```python
from build123d import *

# Parameters (mm, degrees)
SKETCH1_W              = 25.4
SKETCH1_H              = 12.7
BOSS_EXTRUDE1_DEPTH    = 4.7625
F_10_32_TAPPED_HOLE1_D = 4.0386
F_10_32_TAPPED_HOLE2_D = 4.0386


with BuildPart() as part:
    # Sketch1 → Boss-Extrude1 (new, symmetric)
    with BuildSketch(Plane(origin=(0, 0, 0), x_dir=(0, 0, -1), z_dir=(1, 0, 0))):
        Rectangle(SKETCH1_W, SKETCH1_H)
    extrude(amount=BOSS_EXTRUDE1_DEPTH, both=True)

    # #10-32 Tapped Hole1 (through all)
    with Locations(Plane(origin=(0, 6.35, 0), x_dir=(1, 0, 0), z_dir=(0, 1, 0))):
        with Locations((0, 0)):
            Hole(F_10_32_TAPPED_HOLE1_D / 2)

    # #10-32 Tapped Hole2 (through all)
    with Locations(Plane(origin=(4.7625, 0, 0), x_dir=(0, 0, -1), z_dir=(1, 0, 0))):
        with Locations((-7.62, 0), (7.62, 0)):
            Hole(F_10_32_TAPPED_HOLE2_D / 2)


solid = part.part
```
Geometry: final body of the model. Coordinates: model frame, mm. Give positions to 0.01 mm unless a question says otherwise; leave off trailing zeros. Write each loop counter-clockwise with the first axis right and the second up, starting at its lowest first coordinate (ties: lowest second). Pieces come first, ordered by that corner, then holes.
1. Draft query along Y for faces 1 (the flat face through (2.2, -6.35, 0.2)), 2 (the cylindrical face through (-0.067, 0.607, -5.694)), 3 (the flat face through (4.762, 0, 0)). Return one class per face: released by +Y, released by -Y, zero draft, split by the parting line, or undercut.
2. Section query C-C, the plane y = 0. Return loops of the section in (x, z).
3. Section query D-D, the plane z = 7.62. Return loops of the section in (x, y).
4. Line query: probe 1 along Y at (x, z) = (2.25, 7.62); probe 2 along Z at (x, y) = (-1.5, -1); probe 3 along Z at (x, y) = (0, 1). Output: solid intervals per line, ascending.
5. Section query A-A, the plane z = 0. Return loops of the section in (x, y).
6. Section query B-B, the plane x = 0. Return loops of the section in (y, z).
Computed:
1. face 1: released by -Y
1. face 2: undercut
1. face 3: zero draft
2. outline: (-4.76, -12.7) - (4.76, -12.7) - (4.76, -9.64) - (-4.76, -9.64) - close; (-4.76, -5.6) - (4.76, -5.6) - (4.76, 5.6) - (-4.76, 5.6) - close; (-4.76, 9.64) - (4.76, 9.64) - (4.76, 12.7) - (-4.76, 12.7) - close; hole circle Ø4.04 at (0, 0)
3. outline: (-4.76, -6.35) - (4.76, -6.35) - (4.76, -2.02) - (-4.76, -2.02) - close; (-4.76, 2.02) - (4.76, 2.02) - (4.76, 6.35) - (-4.76, 6.35) - close
4. probe 1: y = -6.35 to -2.02, 2.02 to 6.35
4. probe 2: z = -12.7 to -9.37, -5.87 to -1.35, 1.35 to 5.87, 9.37 to 12.7
4. probe 3: z = -12.7 to -9.37, -5.87 to -2.02, 2.02 to 5.87, 9.37 to 12.7
5. outline: (-4.76, -6.35) - (-2.02, -6.35) - (-2.02, 6.35) - (-4.76, 6.35) - close; (2.02, -6.35) - (4.76, -6.35) - (4.76, 6.35) - (2.02, 6.35) - close
6. outline: (-6.35, -12.7) - (6.35, -12.7) - (6.35, -2.02) - (-6.35, -2.02) - close; (-6.35, 2.02) - (6.35, 2.02) - (6.35, 12.7) - (-6.35, 12.7) - close; hole circle Ø4.04 at (0, -7.62); hole circle Ø4.04 at (0, 7.62)
